from build123d import *

# Parameters (mm, degrees)
SKETCH1_W            = 95.5
SKETCH1_H            = 54
BOSS_EXTRUDE1_DEPTH  = 2
SKETCH2_W            = 15
SKETCH2_H            = 2
BOSS_EXTRUDE2_DEPTH  = 2.5
SKETCH3_W            = 15
SKETCH3_H            = 7
BOSS_EXTRUDE3_DEPTH  = 2
CHAMFER1_SIZE        = 3
CUT_EXTRUDE1_REACH   = 59.031
SKETCH4_W            = 10
SKETCH4_H            = 4
BOSS_EXTRUDE4_DEPTH  = 4
FILLET1_R            = 1.901924
FILLET2_R            = 0.2
FILLET1_OF_MIRROR1_R = 1.901924
FILLET2_OF_MIRROR1_R = 0.2
CUT_EXTRUDE5_REACH   = 59.049
SKETCH12_R           = 1.5
SKETCH12_R_2         = 1
CUT_EXTRUDE6_REACH   = 59.049
SKETCH13_W           = 4.8
SKETCH13_H           = 7
CUT_EXTRUDE2_REACH   = 59.317
SKETCH8_W            = 7
SKETCH8_H            = 8.65
BOSS_EXTRUDE5_DEPTH  = 3
CUT_EXTRUDE3_REACH   = 60.049
CUT_EXTRUDE3_START   = 1
SKETCH9_3_R          = 1
SKETCH10_W           = 52.3
SKETCH10_H           = 24.5
SKETCH10_W_2         = 48.3
SKETCH10_H_2         = 20.5
BOSS_EXTRUDE6_DEPTH  = 3
CUT_EXTRUDE4_REACH   = 60.049
CUT_EXTRUDE4_START   = 1
SKETCH10_4_R         = 1.25


with BuildPart() as part:
    # Sketch1 → Boss-Extrude1 (new body)
    with BuildSketch(Plane(origin=(0, 0, 0), x_dir=(1, 0, 0), z_dir=(0, 1, 0))):
        Rectangle(SKETCH1_W, SKETCH1_H)
    extrude(amount=BOSS_EXTRUDE1_DEPTH)

    # Sketch2 → Boss-Extrude2 (add)
    with BuildSketch(Plane.XZ.offset(-2)):
        with Locations((-25, -24.5)):
            Rectangle(SKETCH2_W, SKETCH2_H)
        with Locations((25, -24.5)):
            Rectangle(SKETCH2_W, SKETCH2_H)
    extrude(amount=-BOSS_EXTRUDE2_DEPTH)

    # Sketch3 → Boss-Extrude3 (add)
    with BuildSketch(Plane(origin=(0, 4.5, 0), x_dir=(-1, 0, 0), z_dir=(0, 1, 0))):
        with Locations((-25, -27)):
            Rectangle(SKETCH3_W, SKETCH3_H)
        with Locations((25, -27)):
            Rectangle(SKETCH3_W, SKETCH3_H)
    extrude(amount=BOSS_EXTRUDE3_DEPTH)

    # Chamfer1
    chamfer1_edges = [part.edges().sort_by_distance(p)[0] for p in [
        (32.5, 5.5, -30.5),
        (17.5, 5.5, -30.5),
        (-17.5, 5.5, -30.5),
        (-32.5, 5.5, -30.5),
    ]]
    chamfer(chamfer1_edges, length=CHAMFER1_SIZE)

    # Sketch4 → Cut-Extrude1 (cut, up to next)
    with BuildSketch(Plane.XZ, mode=Mode.PRIVATE) as cut_extrude1_sk1:
        with Locations((-20, 25)):
            Rectangle(SKETCH4_W, SKETCH4_H)
    cut_extrude1_tool1 = extrude(cut_extrude1_sk1.sketch, amount=-CUT_EXTRUDE1_REACH, mode=Mode.PRIVATE) & part.part
    # Sketch4 → Cut-Extrude1 (cut, up to next)
    with BuildSketch(Plane.XZ, mode=Mode.PRIVATE) as cut_extrude1_sk2:
        with Locations((20, 25)):
            Rectangle(SKETCH4_W, SKETCH4_H)
    cut_extrude1_tool2 = extrude(cut_extrude1_sk2.sketch, amount=-CUT_EXTRUDE1_REACH, mode=Mode.PRIVATE) & part.part
    add(cut_extrude1_tool1.solids().sort_by_distance((-20, 0, 25))[0], mode=Mode.SUBTRACT)
    add(cut_extrude1_tool2.solids().sort_by_distance((20, 0, 25))[0], mode=Mode.SUBTRACT)

    # Sketch6 → Boss-Extrude4 (add, symmetric)
    with BuildSketch(Plane(origin=(-20, 0, 0), x_dir=(0, 0, -1), z_dir=(1, 0, 0))):
        Polygon((-21.5, 2), (-21.5, 8.656921938), (-24.5, 8.656921938), (-26, 6.058845727), (-26.9, 4.5), (-26, 4.5), (-26, 0), (-24.5, 0), (-23, 7.656921938), (-23, 2), align=None)
    boss_extrude4 = extrude(amount=BOSS_EXTRUDE4_DEPTH, both=True)

    # Fillet1
    fillet1_edges = [part.edges().sort_by_distance(p)[0] for p in [
        (-20, 8.656921938, 21.5),
        (-20, 8.656921938, 24.5),
    ]]
    fillet(fillet1_edges, radius=FILLET1_R - 0.0001)  # a hair under: the kernel refuses the full size

    # Fillet2
    fillet2_edges = [part.edges().sort_by_distance(p)[0] for p in [
        (-20, 7.656921938, 23),
    ]]
    fillet(fillet2_edges, radius=FILLET2_R)

    # Mirror1: Boss-Extrude4 across plane
    add(boss_extrude4.mirror(Plane(origin=(0, 0, 0), x_dir=(0, 0, 1), z_dir=(1, 0, 0))))

    # Fillet1 of Mirror1
    fillet1_of_mirror1_edges = [part.edges().sort_by_distance(p)[0] for p in [
        (20, 8.656921938, 21.5),
        (20, 8.656921938, 24.5),
    ]]
    fillet(fillet1_of_mirror1_edges, radius=FILLET1_OF_MIRROR1_R - 0.0001)  # a hair under: the kernel refuses the full size

    # Fillet2 of Mirror1
    fillet2_of_mirror1_edges = [part.edges().sort_by_distance(p)[0] for p in [
        (20, 7.656921938, 23),
    ]]
    fillet(fillet2_of_mirror1_edges, radius=FILLET2_OF_MIRROR1_R)

    # Sketch12 → Cut-Extrude5 (cut, up to next)
    with BuildSketch(Plane(origin=(0, 2, 0), x_dir=(1, 0, 0), z_dir=(0, 1, 0)), mode=Mode.PRIVATE) as cut_extrude5_sk1:
        with Locations(Location((2.9867, -20.8641, 0), (0, 0, 270))):
            Circle(SKETCH12_R)
    cut_extrude5_tool1 = extrude(cut_extrude5_sk1.sketch, amount=-CUT_EXTRUDE5_REACH, mode=Mode.PRIVATE) & part.part
    # Sketch12 → Cut-Extrude5 (cut, up to next)
    with BuildSketch(Plane(origin=(0, 2, 0), x_dir=(1, 0, 0), z_dir=(0, 1, 0)), mode=Mode.PRIVATE) as cut_extrude5_sk2:
        with Locations(Location((-44.75, -24, 0), (0, 0, 270))):
            Circle(SKETCH12_R_2)
    cut_extrude5_tool2 = extrude(cut_extrude5_sk2.sketch, amount=-CUT_EXTRUDE5_REACH, mode=Mode.PRIVATE) & part.part
    # Sketch12 → Cut-Extrude5 (cut, up to next)
    with BuildSketch(Plane(origin=(0, 2, 0), x_dir=(1, 0, 0), z_dir=(0, 1, 0)), mode=Mode.PRIVATE) as cut_extrude5_sk3:
        with Locations(Location((44.75, -24, 0), (0, 0, 270))):
            Circle(SKETCH12_R_2)
    cut_extrude5_tool3 = extrude(cut_extrude5_sk3.sketch, amount=-CUT_EXTRUDE5_REACH, mode=Mode.PRIVATE) & part.part
    # Sketch12 → Cut-Extrude5 (cut, up to next)
    with BuildSketch(Plane(origin=(0, 2, 0), x_dir=(1, 0, 0), z_dir=(0, 1, 0)), mode=Mode.PRIVATE) as cut_extrude5_sk4:
        with Locations(Location((-44.75, 24, 0), (0, 0, 270))):
            Circle(SKETCH12_R_2)
    cut_extrude5_tool4 = extrude(cut_extrude5_sk4.sketch, amount=-CUT_EXTRUDE5_REACH, mode=Mode.PRIVATE) & part.part
    # Sketch12 → Cut-Extrude5 (cut, up to next)
    with BuildSketch(Plane(origin=(0, 2, 0), x_dir=(1, 0, 0), z_dir=(0, 1, 0)), mode=Mode.PRIVATE) as cut_extrude5_sk5:
        with Locations(Location((44.75, 24, 0), (0, 0, 270))):
            Circle(SKETCH12_R_2)
    cut_extrude5_tool5 = extrude(cut_extrude5_sk5.sketch, amount=-CUT_EXTRUDE5_REACH, mode=Mode.PRIVATE) & part.part
    add(cut_extrude5_tool1.solids().sort_by_distance((2.9867, 2, 20.8641))[0], mode=Mode.SUBTRACT)
    add(cut_extrude5_tool2.solids().sort_by_distance((-44.75, 2, 24))[0], mode=Mode.SUBTRACT)
    add(cut_extrude5_tool3.solids().sort_by_distance((44.75, 2, 24))[0], mode=Mode.SUBTRACT)
    add(cut_extrude5_tool4.solids().sort_by_distance((-44.75, 2, -24))[0], mode=Mode.SUBTRACT)
    add(cut_extrude5_tool5.solids().sort_by_distance((44.75, 2, -24))[0], mode=Mode.SUBTRACT)

    # Sketch13 → Cut-Extrude6 (cut, up to next)
    with BuildSketch(Plane(origin=(0, 2, 0), x_dir=(1, 0, 0), z_dir=(0, 1, 0)), mode=Mode.PRIVATE) as cut_extrude6_sk1:
        with Locations((30.5407, 15.6841)):
            Rectangle(SKETCH13_W, SKETCH13_H)
    cut_extrude6_tool1 = extrude(cut_extrude6_sk1.sketch, amount=-CUT_EXTRUDE6_REACH, mode=Mode.PRIVATE) & part.part
    add(cut_extrude6_tool1.solids().sort_by_distance((30.5407, 2, -15.6841))[0], mode=Mode.SUBTRACT)

    # Sketch8 → Cut-Extrude2 (cut, up to next)
    with BuildSketch(Plane.XZ, mode=Mode.PRIVATE) as cut_extrude2_sk1:
        with Locations((-29.7, -1.825)):
            Rectangle(SKETCH8_W, SKETCH8_H)
    cut_extrude2_tool1 = extrude(cut_extrude2_sk1.sketch, amount=-CUT_EXTRUDE2_REACH, mode=Mode.PRIVATE) & part.part
    add(cut_extrude2_tool1.solids().sort_by_distance((-29.7, 0, -1.825))[0], mode=Mode.SUBTRACT)

    # Sketch9 → Boss-Extrude5 (add)
    with BuildSketch(Plane(origin=(0, 2, 0), x_dir=(1, 0, 0), z_dir=(0, 1, 0))):
        with BuildLine():
            Line((-45.25, -15.05), (-45.25, -19.85))
            Line((-45.25, -19.85), (-40.45, -19.85))
            Line((-40.45, -19.85), (-40.45, -16.85))
            ThreePointArc((-40.45, -16.85), (-40.977207794, -15.577207794), (-42.25, -15.05))
            Line((-42.25, -15.05), (-45.25, -15.05))
        make_face()
        with BuildLine():
            Line((-15.65, -15.05), (-18.65, -15.05))
            ThreePointArc((-18.65, -15.05), (-19.922792206, -15.577207794), (-20.45, -16.85))
            Line((-20.45, -16.85), (-20.45, -19.85))
            Line((-20.45, -19.85), (-15.65, -19.85))
            Line((-15.65, -19.85), (-15.65, -15.05))
        make_face()
        with BuildLine():
            Line((-45.25, 17.05), (-42.25, 17.05))
            ThreePointArc((-42.25, 17.05), (-40.977207794, 17.577207794), (-40.45, 18.85))
            Line((-40.45, 18.85), (-40.45, 21.85))
            Line((-40.45, 21.85), (-45.25, 21.85))
            Line((-45.25, 21.85), (-45.25, 17.05))
        make_face()
        with BuildLine():
            Line((-15.65, 17.05), (-15.65, 21.85))
            Line((-15.65, 21.85), (-20.45, 21.85))
            Line((-20.45, 21.85), (-20.45, 18.85))
            ThreePointArc((-20.45, 18.85), (-19.922792206, 17.577207794), (-18.65, 17.05))
            Line((-18.65, 17.05), (-15.65, 17.05))
        make_face()
    extrude(amount=BOSS_EXTRUDE5_DEPTH)

    # Sketch9<3> → Cut-Extrude3 (cut, up to next)
    with BuildSketch(Plane(origin=(0, 2, 0), x_dir=(1, 0, 0), z_dir=(0, 1, 0)).offset(CUT_EXTRUDE3_START), mode=Mode.PRIVATE) as cut_extrude3_sk1:
        with Locations(Location((-42.25, -16.85, 0), (0, 0, 270))):
            Circle(SKETCH9_3_R)
    cut_extrude3_tool1 = extrude(cut_extrude3_sk1.sketch, amount=CUT_EXTRUDE3_REACH, mode=Mode.PRIVATE) & part.part
    # Sketch9<3> → Cut-Extrude3 (cut, up to next)
    with BuildSketch(Plane(origin=(0, 2, 0), x_dir=(1, 0, 0), z_dir=(0, 1, 0)).offset(CUT_EXTRUDE3_START), mode=Mode.PRIVATE) as cut_extrude3_sk2:
        with Locations(Location((-18.65, -16.85, 0), (0, 0, 90))):
            Circle(SKETCH9_3_R)
    cut_extrude3_tool2 = extrude(cut_extrude3_sk2.sketch, amount=CUT_EXTRUDE3_REACH, mode=Mode.PRIVATE) & part.part
    # Sketch9<3> → Cut-Extrude3 (cut, up to next)
    with BuildSketch(Plane(origin=(0, 2, 0), x_dir=(1, 0, 0), z_dir=(0, 1, 0)).offset(CUT_EXTRUDE3_START), mode=Mode.PRIVATE) as cut_extrude3_sk3:
        with Locations(Location((-42.25, 18.85, 0), (0, 0, 90))):
            Circle(SKETCH9_3_R)
    cut_extrude3_tool3 = extrude(cut_extrude3_sk3.sketch, amount=CUT_EXTRUDE3_REACH, mode=Mode.PRIVATE) & part.part
    # Sketch9<3> → Cut-Extrude3 (cut, up to next)
    with BuildSketch(Plane(origin=(0, 2, 0), x_dir=(1, 0, 0), z_dir=(0, 1, 0)).offset(CUT_EXTRUDE3_START), mode=Mode.PRIVATE) as cut_extrude3_sk4:
        with Locations(Location((-18.65, 18.85, 0), (0, 0, 270))):
            Circle(SKETCH9_3_R)
    cut_extrude3_tool4 = extrude(cut_extrude3_sk4.sketch, amount=CUT_EXTRUDE3_REACH, mode=Mode.PRIVATE) & part.part
    add(cut_extrude3_tool1.solids().sort_by_distance((-42.25, 3, 16.85))[0], mode=Mode.SUBTRACT)
    add(cut_extrude3_tool2.solids().sort_by_distance((-18.65, 3, 16.85))[0], mode=Mode.SUBTRACT)
    add(cut_extrude3_tool3.solids().sort_by_distance((-42.25, 3, -18.85))[0], mode=Mode.SUBTRACT)
    add(cut_extrude3_tool4.solids().sort_by_distance((-18.65, 3, -18.85))[0], mode=Mode.SUBTRACT)

    # Sketch10 → Boss-Extrude6 (add)
    # profile 1 of 2: a face of its own
    with BuildSketch(Plane(origin=(0, 2, 0), x_dir=(1, 0, 0), z_dir=(0, 1, 0))):
        with Locations((18.6, -4.75)):
            Rectangle(SKETCH10_W, SKETCH10_H)
        with Locations((18.6, -4.75)):
            Rectangle(SKETCH10_W_2, SKETCH10_H_2, mode=Mode.SUBTRACT)
    # profile 2 of 2: a face of its own
    with BuildSketch(Plane(origin=(0, 2, 0), x_dir=(1, 0, 0), z_dir=(0, 1, 0))):
        with BuildLine():
            Line((4.134296709, 0.955780252), (34.134296709, -4.044219748))
            ThreePointArc((34.134296709, -4.044219748), (36.805780252, -7.784296709), (33.065703291, -10.455780252))
            Line((33.065703291, -10.455780252), (3.065703291, -5.455780252))
            ThreePointArc((3.065703291, -5.455780252), (0.394219748, -1.715703291), (4.134296709, 0.955780252))
        make_face()
    extrude(amount=BOSS_EXTRUDE6_DEPTH)

    # Sketch10<4> → Cut-Extrude4 (cut, up to next)
    with BuildSketch(Plane(origin=(0, 2, 0), x_dir=(1, 0, 0), z_dir=(0, 1, 0)).offset(CUT_EXTRUDE4_START), mode=Mode.PRIVATE) as cut_extrude4_sk1:
        with Locations(Location((18.6, -4.75, 0), (0, 0, 270))):
            Circle(SKETCH10_4_R)
    cut_extrude4_tool1 = extrude(cut_extrude4_sk1.sketch, amount=CUT_EXTRUDE4_REACH, mode=Mode.PRIVATE) & part.part
    # Sketch10<4> → Cut-Extrude4 (cut, up to next)
    with BuildSketch(Plane(origin=(0, 2, 0), x_dir=(1, 0, 0), z_dir=(0, 1, 0)).offset(CUT_EXTRUDE4_START), mode=Mode.PRIVATE) as cut_extrude4_sk2:
        with Locations(Location((3.6, -2.25, 0), (0, 0, 270))):
            Circle(SKETCH10_4_R)
    cut_extrude4_tool2 = extrude(cut_extrude4_sk2.sketch, amount=CUT_EXTRUDE4_REACH, mode=Mode.PRIVATE) & part.part
    # Sketch10<4> → Cut-Extrude4 (cut, up to next)
    with BuildSketch(Plane(origin=(0, 2, 0), x_dir=(1, 0, 0), z_dir=(0, 1, 0)).offset(CUT_EXTRUDE4_START), mode=Mode.PRIVATE) as cut_extrude4_sk3:
        with Locations(Location((33.6, -7.25, 0), (0, 0, 270))):
            Circle(SKETCH10_4_R)
    cut_extrude4_tool3 = extrude(cut_extrude4_sk3.sketch, amount=CUT_EXTRUDE4_REACH, mode=Mode.PRIVATE) & part.part
    add(cut_extrude4_tool1.solids().sort_by_distance((18.6, 3, 4.75))[0], mode=Mode.SUBTRACT)
    add(cut_extrude4_tool2.solids().sort_by_distance((3.6, 3, 2.25))[0], mode=Mode.SUBTRACT)
    add(cut_extrude4_tool3.solids().sort_by_distance((33.6, 3, 7.25))[0], mode=Mode.SUBTRACT)


solid = part.part
For this review, take the finished solid that the model builds, in its own axes (mm). A direction names the side the tool comes from. Give positions to 0.01 mm unless a question says otherwise; leave off trailing zeros. Loops run counter-clockwise (first coordinate to the right, second up) from the corner with the lowest first, then second, coordinate; pieces in that order, holes last.
Item 1: Take a section at D-D, the plane z = 7.25. State the section outline as (x, y) points.
Item 2: For line 1 along X through (y, z) = (4, -19); line 2 along X through (y, z) = (1.4, 24); line 3 along X through (y, z) = (3.8, -18.85), list the stretches that pass through material, from the lowest coordinate up.
Item 3: Take a section at C-C, the plane x = -1. State the section outline as (y, z) points.
Item 4: Take a section at A-A, the plane x = 31. State the section outline as (y, z) points.
Item 5: Draft analysis for pull direction Z (two halves, no side actions). For faces 1 (the flat face through (-15.65, 3, 17)), 2 (the flat face through (-31, 5, -29)), 3 (the flat face through (32.941, 1, -16)), state which applies: +Z half, -Z half, draft (parallel to the pull), parting line (faces both ways), or undercut.
Item 6: Take a section at B-B, the plane z = 13.5. State the section outline as (x, y) points, and give its area (3 significant figures).
Item 7: Insertion check: pin 1 (3.5 mm diameter, centred on x = 20, y = 4, fed in from +Z); pin 2 (0.9 mm diameter, centred on x = -19, y = 4, fed in from -Z); pin 3 (1.5 mm diameter, centred on y = 4, z = 0, fed in from -X); pin 4 (3.5 mm diameter, centred on y = 3, z = 17.5, fed in from +X). Each pin has a flat end and moves straight along its axis. Give the tip position at first contact, or say it passes through.
Item 8: Tool access review of faces 4 (the flat face through (-18, 3, 19.85)), 5 (the flat face through (19, 5, -29)), 6 (the cylindrical face through (-41.26, 3.99, 16.72)), 7 (the flat face through (16, 5, 24)): name each direction out of +Z, -Z, +X, -X, +Y, -Y from which nothing blocks a thin tool from reaching the whole face with its end or side.
Calculated:
1. outline: (-47.75, 0) - (47.75, 0) - (47.75, 2) - (44.75, 2) - (44.75, 5) - (42.75, 5) - (42.75, 2) - (36.85, 2) - (36.85, 5) - (34.85, 5) - (34.85, 3) - (32.35, 3) - (32.35, 5) - (13.83, 5) - (13.83, 2) - (-5.55, 2) - (-5.55, 5) - (-7.55, 5) - (-7.55, 2) - (-47.75, 2) - close
2. line 1: x = -45.25 to -43.24, -41.26 to -40.45, -20.45 to -19.64, -17.66 to -15.65
2. line 2: x = -47.75 to -45.75, -43.75 to -25, -15 to 15, 25 to 43.75, 45.75 to 47.75
2. line 3: x = -45.25 to -43.25, -41.25 to -40.45, -20.45 to -19.65, -17.65 to -15.65
3. outline: (0, -27) - (2, -27) - (2, -7.5) - (5, -7.5) - (5, -5.5) - (2, -5.5) - (2, 15) - (5, 15) - (5, 17) - (2, 17) - (2, 27) - (0, 27) - close
4. outline: (0, -27) - (2, -27) - (2, -25.5) - (4.5, -25.5) - (4.5, -29) - (6.5, -29) - (6.5, -23.5) - (2, -23.5) - (2, -19.18) - (0, -19.18) - close; (0, -12.18) - (2, -12.18) - (2, -7.5) - (5, -7.5) - (5, -5.5) - (2, -5.5) - (2, 3.52) - (5, 3.52) - (5, 10.11) - (2, 10.11) - (2, 15) - (5, 15) - (5, 17) - (2, 17) - (2, 27) - (0, 27) - close
5. face 1: draft
5. face 2: -Z half
5. face 3: undercut
6. outline: (-47.75, 0) - (47.75, 0) - (47.75, 2) - (44.75, 2) - (44.75, 5) - (42.75, 5) - (42.75, 2) - (-5.55, 2) - (-5.55, 5) - (-7.55, 5) - (-7.55, 2) - (-47.75, 2) - close
6. area: 203 mm2
7. pin 1: stops at z = 26.9
7. pin 2: stops at z = -25.5
7. pin 3: stops at x = -7.55
7. pin 4: stops at x = 47.75
8. face 4: +X, -X, +Y
8. face 5: -Z, +Y, -Y
8. face 6: +Y
8. face 7: +Z, +Y
